Work out the finished part from the listing and answer in its coordinate system (mm). A direction names the side the tool comes from. Round coordinates to 2 decimals unless told otherwise and drop trailing zeros. Loops run counter-clockwise (first coordinate to the right, second up) from the corner with the lowest first, then second, coordinate; pieces in that order, holes last.
```python
from build123d import *

# Parameters (mm, degrees)
BOSS_EXTRUDE1_REACH      = 48.609
BOSS_EXTRUDE1_END_RADIUS = 11.2014
SKETCH2_W                = 1.3462
SKETCH2_H                = 4.4704


with BuildPart() as part:
    # Sketch1 → Revolve1 (revolve)
    with BuildSketch(Plane.XY):
        Polygon((-11.2014, 18.161), (-11.2014, 0), (0, 0), (0, 38.9382), (-3.1242, 38.9382), (-3.1242, 27.1272), (-4.6355, 27.1272), (-4.6355, 19.7612), (-5.0546, 19.7612), (-5.0546, 18.161), align=None)
    revolve(axis=Axis((0, 0, 0), (0, -1, 0)))

    # Boss-Extrude1: up to this cylinder (the profile starts outside it)
    boss_extrude1_end = Plane(origin=(0, 9.0805, 0), z_dir=(0, 1, 0)) * Cylinder(BOSS_EXTRUDE1_END_RADIUS, 134.3114, mode=Mode.PRIVATE)
    # Sketch2 → Boss-Extrude1 (add, up to the surface)
    with BuildSketch(Plane(origin=(11.8364, 0, 0), x_dir=(0, 0, -1), z_dir=(1, 0, 0)), mode=Mode.PRIVATE) as boss_extrude1_sk1:
        with Locations((-5.3975, 15.9258)):
            Rectangle(SKETCH2_W, SKETCH2_H)
    boss_extrude1_tool1 = extrude(boss_extrude1_sk1.sketch, amount=-BOSS_EXTRUDE1_REACH, mode=Mode.PRIVATE) - boss_extrude1_end
    # Sketch2 → Boss-Extrude1 (add, up to the surface)
    with BuildSketch(Plane(origin=(11.8364, 0, 0), x_dir=(0, 0, -1), z_dir=(1, 0, 0)), mode=Mode.PRIVATE) as boss_extrude1_sk2:
        with Locations((-5.3975, 2.2352)):
            Rectangle(SKETCH2_W, SKETCH2_H)
    boss_extrude1_tool2 = extrude(boss_extrude1_sk2.sketch, amount=-BOSS_EXTRUDE1_REACH, mode=Mode.PRIVATE) - boss_extrude1_end
    boss_extrude1 = boss_extrude1_tool1.solids().sort_by_distance((11.8364, 15.9258, 5.3975))[0] + boss_extrude1_tool2.solids().sort_by_distance((11.8364, 2.2352, 5.3975))[0]
    add(boss_extrude1)

    # Mirror1: Boss-Extrude1 across plane
    add(boss_extrude1.mirror(Plane.XY))


solid = part.part
```
1. Determine the mould class of faces 6 (the face through (5.3, 18.161, -0.2)), 7 (the face through (11, 13.691, 5)), 8 (the face through (11, 13.691, -5)), 9 (the face through (-2.98, 32.95, -0.94)) for opening direction Y: +Y half, -Y half, draft (parallel to the pull), parting line (faces both ways), or undercut.
Answer key:
face 6: +Y half
face 7: undercut
face 8: undercut
face 9: draft
2. Given pin 1 (1.8 mm diameter, centred on x = 11, y = 1, fed in from -Z); pin 2 (1.8 mm diameter, centred on x = 10.5, y = 15, fed in from +Z); pin 3 (0.7 mm diameter, centred on x = 10.5, z = -5.5, fed in from -Y); pin 4 (3 mm diameter, centred on y = 26.5, z = -7, fed in from +X), each flat-ended and moving along its own axis, determine where each tip first touches the part or whether it passes through.
Answer key:
pin 1: stops at z = -6.07
pin 2: stops at z = 6.07
pin 3: stops at y = 0
pin 4: passes through
3. Find section B-B (x = 0). Write down the section's boundary in (y, z), then the cut area to 3 significant figures.
Answer key:
outline: (0, -11.2) - (18.16, -11.2) - (18.16, -5.05) - (19.76, -5.05) - (19.76, -4.64) - (27.13, -4.64) - (27.13, -3.12) - (38.94, -3.12) - (38.94, 3.12) - (27.13, 3.12) - (27.13, 4.64) - (19.76, 4.64) - (19.76, 5.05) - (18.16, 5.05) - (18.16, 11.2) - (0, 11.2) - close
area: 565 mm2
4. Consider probe 1 along Y at (x, z) = (10, 5.75); probe 2 along Y at (x, z) = (7, 6); probe 3 along X at (y, z) = (14, 0). Determine where each line is inside the solid, lowest interval first.
Answer key:
probe 1: y = 0 to 4.47, 13.69 to 18.16
probe 2: y = 0 to 18.16
probe 3: x = -11.2 to 11.2
5. Find section C-C (y = 7). Write down the section's boundary in (x, z).
Answer key:
outline: circle Ø22.4 at (0, 0)
6. Find section D-D (z = 8.75). Write down the section's boundary in (x, y), then the cut area to 3 significant figures.
Answer key:
outline: (-6.99, 0) - (6.99, 0) - (6.99, 18.16) - (-6.99, 18.16) - close
area: 254 mm2
7. Which of the six approach directions +Z, -Z, +X, -X, +Y, -Y give full straight-line access (tool end or side, diameter ignored) to faces 1 (the face through (11.836, 2, -5)), 2 (the face through (11, 2, 4.724)), 3 (the face through (11, 16, 6.071)), 4 (the face through (3.42, 23.39, -3.13)), 5 (the face through (11, 2, -6.071))?
Answer key:
face 1: +Z, -Z, +X, +Y, -Y
face 2: +X, +Y, -Y
face 3: +Z, +X, +Y, -Y
face 4: +Y
face 5: -Z, +X, +Y, -Y
8. Find section A-A (z = 0). Write down the section's boundary in (x, y).
Answer key:
outline: (-11.2, 0) - (11.2, 0) - (11.2, 18.16) - (5.05, 18.16) - (5.05, 19.76) - (4.64, 19.76) - (4.64, 27.13) - (3.12, 27.13) - (3.12, 38.94) - (-3.12, 38.94) - (-3.12, 27.13) - (-4.64, 27.13) - (-4.64, 19.76) - (-5.05, 19.76) - (-5.05, 18.16) - (-11.2, 18.16) - close
